Geometry: final body of the model. Coordinates: model frame, mm. Face numbers are marked on the shaded views. A direction names the side the tool comes from. Give positions to 0.01 mm unless a question says otherwise; leave off trailing zeros. Write each loop counter-clockwise with the first axis right and the second up, starting at its lowest first coordinate (ties: lowest second). Pieces come first, ordered by that corner, then holes.
```python
from build123d import *

# Parameters (mm, degrees)
SKETCH_1_R      = 2
EXTRUDE_1_DEPTH = 1.1


with BuildPart() as part:
    # 草图1 → 凸台-拉伸1 (new body)
    with BuildSketch(Plane(origin=(0, 0, 0), x_dir=(1, 0, 0), z_dir=(0, 1, 0))):
        with BuildLine():
            Line((-9.955555556, 12.525450634), (-23.744444444, 1.565681329))
            ThreePointArc((-23.744444444, 1.565681329), (-24.5, 0), (-23.744444444, -1.565681329))
            Line((-23.744444444, -1.565681329), (-9.955555556, -12.525450634))
            ThreePointArc((-9.955555556, -12.525450634), (0, -16), (9.955555556, -12.525450634))
            Line((9.955555556, -12.525450634), (23.744444444, -1.565681329))
            ThreePointArc((23.744444444, -1.565681329), (24.5, 0), (23.744444444, 1.565681329))
            Line((23.744444444, 1.565681329), (9.955555556, 12.525450634))
            ThreePointArc((9.955555556, 12.525450634), (0, 16), (-9.955555556, 12.525450634))
        make_face()
        with Locations((-19, 0)):
            Circle(SKETCH_1_R, mode=Mode.SUBTRACT)
        with Locations((19, 0)):
            Circle(SKETCH_1_R, mode=Mode.SUBTRACT)
    extrude(amount=EXTRUDE_1_DEPTH)

    # 草图2 → 旋转1 (revolve)
    with BuildSketch(Plane.XY):
        with BuildLine():
            Line((0, 1.1), (-13.5, 1.1))
            Line((-13.5, 1.1), (-13.5, 13))
            ThreePointArc((-13.5, 13), (-12.621320344, 15.121320344), (-10.5, 16))
            Line((-10.5, 16), (-7.348469228, 16))
            ThreePointArc((-7.348469228, 16), (-4.444097209, 19.631462317), (0, 21))
            Line((0, 21), (0, 1.1))
        make_face()
    revolve(axis=Axis((0, 1.1, 0), (0, 1, 0)))


solid = part.part
```
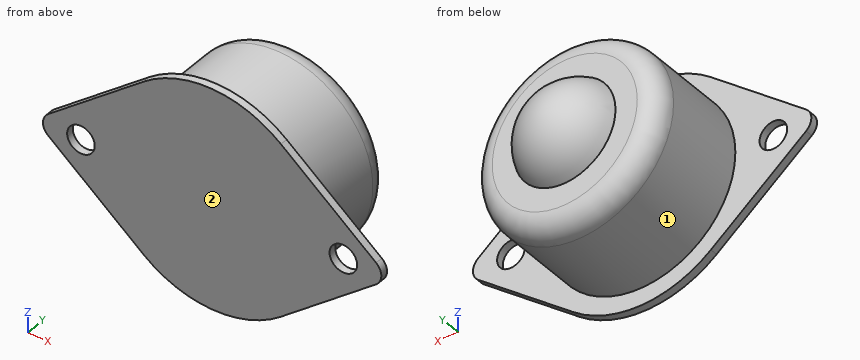
Item 1: Section C-C, the plane y = 4.5. Return the cut outline in (x, z), plus the area to 3 significant figures.
Found:
outline: circle Ø27 at (0, 0)
area: 573 mm2
Item 2: Pin query (flat end, axial travel): pin 1 Ø1.5 at (x, z) = (-11.5, -7) entering from +Y; pin 2 Ø3 at (y, z) = (12.5, 9.5) entering from +X; pin 3 Ø1.5 at (x, z) = (-1.5, 5.5) entering from +Y; pin 4 Ø3.5 at (x, z) = (19, 0) entering from +Y. Return the tip coordinate at first contact, or that it passes through.
Found:
pin 1: stops at y = 15.03
pin 2: stops at x = 10.87
pin 3: stops at y = 19.26
pin 4: passes through
Item 3: Section B-B, the plane x = 17.5. Return the cut outline in (y, z), plus the area to 3 significant figures.
Found:
outline: (0, -6.53) - (1.1, -6.53) - (1.1, -1.32) - (0, -1.32) - close; (0, 1.32) - (1.1, 1.32) - (1.1, 6.53) - (0, 6.53) - close
area: 11.5 mm2
Item 4: Reachability of the marked faces 1 and 2 from +Z, -Z, +X, -X, +Y, -Y: full face, straight path, thin tool, end or side. Return the list, or none.
Found:
face 1: +Y
face 2: +Z, -Z, +X, -X, -Y
Item 5: Line query: L1, parallel to Y at x = -15, z = -7.5; L2, parallel to Z at x = 19, y = 0.55; L3, parallel to Z at x = -0.5, y = 1.75. Output: solid intervals per line, ascending.
Found:
L1: y = 0 to 1.1
L2: z = -5.34 to -2, 2 to 5.34
L3: z = -13.49 to 13.49
Item 6: Section A-A, the plane z = 0. Return the cut outline in (x, y).
Found:
outline: (-24.5, 0) - (-21, 0) - (-21, 1.1) - (-24.5, 1.1) - close; (-17, 0) - (17, 0) - (17, 1.1) - (13.5, 1.1) - (13.5, 13) arc R3 ccw to (10.5, 16) - (7.35, 16) arc R7.9 ccw to (-7.35, 16) - (-10.5, 16) arc R3 ccw to (-13.5, 13) - (-13.5, 1.1) - (-17, 1.1) - close; (21, 0) - (24.5, 0) - (24.5, 1.1) - (21, 1.1) - close
Item 7: Section D-D, the plane x = -16. Return the cut outline in (y, z), plus the area to 3 significant figures.
Found:
outline: (0, -7.72) - (1.1, -7.72) - (1.1, 7.72) - (0, 7.72) - close
area: 17.0 mm2
